The model under review builds one solid part; all positions refer to its coordinate system, in mm. Face numbers are marked on the shaded views. Coordinates: 2 decimals unless noted, no trailing zeros. Order: outer loops, then holes, each group sorted by start corner. A loop starts at its lowest first (then second) coordinate and runs counter-clockwise, first axis right, second up. Notation, with made-up numbers: (57.25, 42) -> (114.25, 42) arc R28 ccw to (114.25, 70) -> close; hole circle Ø11 at (37, -32.75). An arc over 180 degrees is marked (long way). Use one line per item in the form item = value. Start each with the question number.
(1) Insertion check: pin 1 Ø22.5 at (x, z) = (46.5, -25.5) entering from -Y; pin 2 Ø2.5 at (x, z) = (86.5, -3.5) entering from -Y; pin 3 Ø2.5 at (x, z) = (1.5, -15) entering from -Y. Each pin has a flat end and moves straight along its axis. Give the tip position at first contact, or say it passes through.
(2) Mouldability with a two-part tool opening along Z and no side actions: class the marked faces 1, 2 and 3 as +Z half, -Z half, draft (parallel to the pull), parting line (faces both ways), or undercut.
(3) Wall thickness on line 1 along Z through (x, y) = (49, -5.5); line 2 along X through (y, z) = (-9.25, -30); line 3 along Y through (x, z) = (67, -38): over which ranges is each line inside the solid? List them lowest first.
(4) Take a section at B-B (x = 78.5). State the section outline as (y, z) points.
(5) Take a section at A-A (y = -8.5). State the section outline as (x, z) points.
(6) Take a section at C-C (z = -39). State the section outline as (x, y) points.
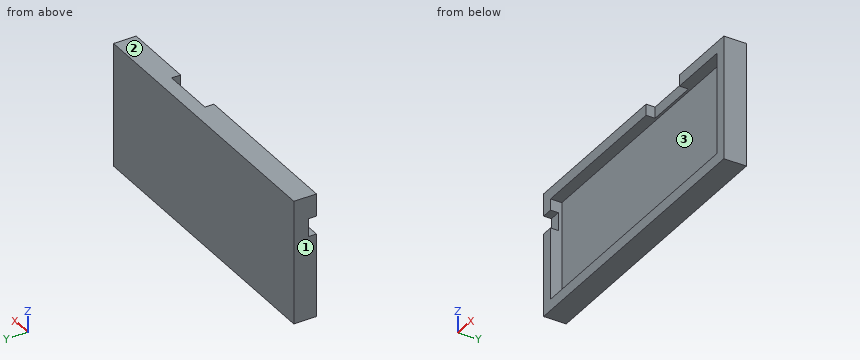
```python
from build123d import *

# Parameters (mm, degrees)
F0_W     = 130
F0_H     = 55
F1_DEPTH = 10
F2_T     = -5
F4_DEPTH = 11.684
F5_W     = 3.5
F5_H     = 8
F6_DEPTH = 6.7818


with BuildPart() as f1:
    # F0 (on Front) → F1 (new body)
    with BuildSketch(Plane.XZ):
        with Locations((65, -27.5)):
            Rectangle(F0_W, F0_H)
    extrude(amount=F1_DEPTH)

    # F2
    f2_openings = [f1.faces().sort_by_distance(p)[0] for p in [
        (65, -10, -27.5),
    ]]
    offset(amount=F2_T, openings=f2_openings)

    # F3 (on Top) → F4 (cut)
    with BuildSketch(Plane.XY):
        Polygon((73.914569, -6.014053), (73.914569, -10.014053), (97.914569, -10.014053), (97.914569, -9.998512), (97.914569, -6.014053), align=None)
    extrude(amount=-F4_DEPTH, mode=Mode.SUBTRACT)

    # F5 (on Right) → F6 (cut)
    with BuildSketch(Plane.YZ):
        with Locations((-8.289312, -14.001081)):
            Rectangle(F5_W, F5_H)
    extrude(amount=F6_DEPTH, mode=Mode.SUBTRACT)


solid = f1.part
```
Findings:
q1.pin_1 = -5
q1.pin_2 = -6.01
q1.pin_3 = -6.54
q2.face_1 = draft
q2.face_2 = +Z half
q2.face_3 = undercut
q3.line_1 = -55 to -50, -5 to 0
q3.line_2 = 0 to 5, 125 to 130
q3.line_3 = -5 to 0
q4.outline = (-10, -55) -> (0, -55) -> (0, 0) -> (-6.01, 0) -> (-6.01, -5) -> (-5, -5) -> (-5, -50) -> (-10, -50) -> close
q5.outline = (0, -55) -> (130, -55) -> (130, 0) -> (97.91, 0) -> (97.91, -5) -> (125, -5) -> (125, -50) -> (5, -50) -> (5, -18) -> (0, -18) -> close; (0, -10) -> (5, -10) -> (5, -5) -> (73.91, -5) -> (73.91, 0) -> (0, 0) -> close
q6.outline = (0, -10) -> (5, -10) -> (5, -5) -> (125, -5) -> (125, -10) -> (130, -10) -> (130, 0) -> (0, 0) -> close
